```python
from build123d import *

# Parameters (mm, degrees)
SKETCH1_R                                          = 100.375000037
SKETCH1_R_2                                        = 85.74999995
BOSS_EXTRUDE1_DEPTH                                = 5.000000033
SKETCH2_R                                          = 1.27
CUT_EXTRUDE1_DEPTH                                 = 143.03971721
CIRPATTERN1_COUNT                                  = 4
CSK_FOR_10_FLAT_HEAD_MACHINE_SCREW_100_D           = 5.1054
CSK_FOR_10_FLAT_HEAD_MACHINE_SCREW_100_CSINK_D     = 9.779
CSK_FOR_10_FLAT_HEAD_MACHINE_SCREW_100_CSINK_ANGLE = 100


with BuildPart() as part:
    # Sketch1 → Boss-Extrude1 (new, symmetric)
    with BuildSketch(Plane(origin=(0, 0, 0), x_dir=(1, 0, 0), z_dir=(0, 1, 0))):
        with Locations(Location((0, 0, 0), (0, 0, 270))):
            Circle(SKETCH1_R)
        with Locations(Location((0, 0, 0), (0, 0, 270))):
            Circle(SKETCH1_R_2, mode=Mode.SUBTRACT)
    extrude(amount=BOSS_EXTRUDE1_DEPTH, both=True)

    # Sketch2 → Cut-Extrude1 (cut, symmetric)
    with BuildSketch(Plane(origin=(0, 0, 0), x_dir=(1, 0, 0), z_dir=(0, 1, 0))):
        with Locations(Location((-93.125000059, 0, 0), (0, 0, 270))):
            Circle(SKETCH2_R)
    cut_extrude1 = extrude(amount=CUT_EXTRUDE1_DEPTH, both=True, mode=Mode.SUBTRACT)

    # CirPattern1: Cut-Extrude1 ×4 about axis
    cirpattern1_axis = Axis((0, 0, 0), (0, 1, 0))
    for i in range(1, CIRPATTERN1_COUNT):
        add(cut_extrude1.rotate(cirpattern1_axis, i * 360 / CIRPATTERN1_COUNT), mode=Mode.SUBTRACT)

    # CSK for #10 Flat Head Machine Screw (100)1 (through all)
    with Locations(Plane(origin=(93.125000059, -5.000000033, 0), x_dir=(0, 0, -1), z_dir=(0, -1, 0))):
        with Locations((0, 0), (93.125000059, -93.125000059), (0, -186.250000118), (-93.125000059, -93.125000059)):
            CounterSinkHole(CSK_FOR_10_FLAT_HEAD_MACHINE_SCREW_100_D / 2, CSK_FOR_10_FLAT_HEAD_MACHINE_SCREW_100_CSINK_D / 2, counter_sink_angle=CSK_FOR_10_FLAT_HEAD_MACHINE_SCREW_100_CSINK_ANGLE)


solid = part.part
```
The listing builds one solid part. Answer for the finished solid, in the listing's coordinates (mm). Coordinates: 2 decimals unless noted, no trailing zeros. Write each loop counter-clockwise with the first axis right and the second up, starting at its lowest first coordinate (ties: lowest second). Pieces come first, ordered by that corner, then holes. Notation, with made-up numbers: (41.25, -32.5) - (99.25, -32.5) arc R20 cw to (99.25, -16.5) - close; hole circle Ø11 at (35.5, 32.25). An arc over 180 degrees is marked (long way). One line per item, written item: value.
1) Each of these flat-tipped pins is pushed along its axis until it touches: pin 1 Ø6.5 at (x, z) = (93.125, 0) entering from -Y; pin 2 Ø5 at (x, y) = (-22.5, -1.5) entering from -Z; pin 3 Ø1.5 at (y, z) = (0, -16) entering from -X. Where does it stop, or does it pass through?
Geometry check:
pin 1: stops at y = -3.62
pin 2: stops at z = -98.36
pin 3: stops at x = -99.21
2) Find section A-A (z = 0). Count the separate pieces of the cut face and the enclosed holes in it, and give its area (3 significant figures).
Geometry check:
separate pieces: 4
enclosed holes: 0
area: 181 mm2
3) Consider line 1 along X through (y, z) = (-0.5, 0) (3 decimals); line 2 along X through (y, z) = (3.5, 42.5); line 3 along X through (y, z) = (1, 34). Determine where each line is inside the solid, lowest interval first. Write a range as from..to.
Geometry check:
line 1: x = -100.375..-95.678, -90.572..-85.75, 85.75..90.572, 95.678..100.375
line 2: x = -90.93..-74.48, 74.48..90.93
line 3: x = -94.44..-78.72, 78.72..94.44
4) Find section D-D (z = -46). Give the vertices of the cut face in (x, y).
Geometry check:
outline: (-89.21, -5) - (-72.37, -5) - (-72.37, 5) - (-89.21, 5) - close; (72.37, -5) - (89.21, -5) - (89.21, 5) - (72.37, 5) - close
5) For a pull along Z with two mould halves and no side action, classify faces 1 (the flat face through (75, -5, 44)), 2 (the cylindrical face through (-83.71, -0.07, -18.59)), 3 (the cylindrical face through (99.52, 0.07, -13.07)) as pulls with the +Z half, pulls with the -Z half, needs draft (parallel to the pull), parting line crosses it, or undercut.
Geometry check:
face 1: needs draft
face 2: undercut
face 3: parting line crosses it
6) Find section C-C (x = -68). Give the vertices of the cut face in (y, z).
Geometry check:
outline: (-5, -73.83) - (5, -73.83) - (5, -52.24) - (-5, -52.24) - close; (-5, 52.24) - (5, 52.24) - (5, 73.83) - (-5, 73.83) - close
